Can you work these out from the model? Positions are in its coordinate system, mm. Coordinates: 2 decimals unless noted, no trailing zeros. Loops run counter-clockwise (first coordinate to the right, second up) from the corner with the lowest first, then second, coordinate; pieces in that order, holes last.
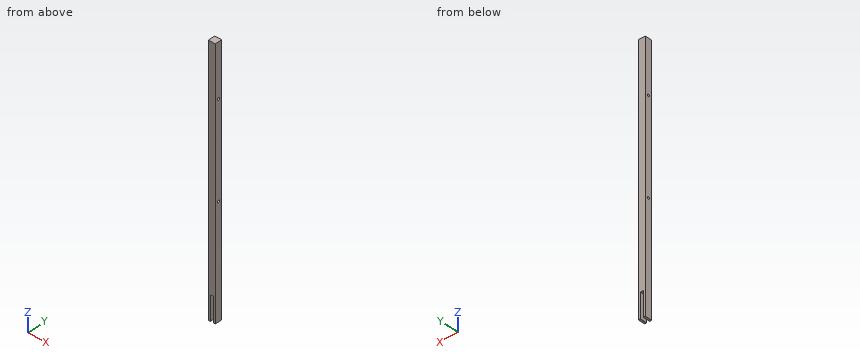
Autodesk Inventor part; units mm, degrees
ref_plane "YZ Plane" through (0, 0, 0) normal (1, 0, 0) x (0, 1, 0)
ref_plane "XZ Plane" through (0, 0, 0) normal (0, 1, 0) x (-1, 0, 0)
ref_plane "XY Plane" through (0, 0, 0) normal (0, 0, 1) x (1, 0, 0)
sketch "Sketch1" plane through (0, 0, 0) normal (0, 0, 1) x (1, 0, 0)
  line L0 (-6, -6) -> (6, -6)
  line L1 (6, -6) -> (6, 6)
  line L2 (6, 6) -> (-6, 6)
  line L3 (-6, 6) -> (-6, -6)
  line L4 (-6, -6) -> (6, 6) construction
  line L5 (6, -6) -> (-6, 6) construction
  point P0 (0, 0)
  dimension "d0" = 12
  dimension "d1" = 12
extrude "Extrusion1" add sketch "Sketch1" along normal blind 440
sketch "Sketch4" plane through (-6, 6, 0) normal (0, 1, 0) x (1, 0, 0)
  line L0 (12, 0) -> (0, 0)
  line L1 (0, 0) -> (0, -440)
  line L2 (12, -440) -> (0, -440)
  line L3 (12, 0) -> (12, -440)
  line L4 (3.5, 0) -> (3.5, -42)
  line L5 (3.5, -42) -> (8.5, -42)
  line L6 (8.5, -42) -> (8.5, 0)
  point P0 (6, 0)
  point P1 (6, -42)
  point P2 (6, 0)
  dimension "d17" = 5
  dimension "d18" = 42
extrude "Extrusion3" cut sketch "Sketch4" against normal through all contours L6 L5 L4 L0
sketch "Sketch5" plane through (6, -6, 0) normal (1, 0, 0) x (0, 0, -1)
  line L0 (-440, 0) -> (-440, 12)
  point P0 (0, 6)
  point P1 (-350, 6)
  point P2 (-189, 6)
  point P3 (-440, 6)
  dimension "d21" = 161
  dimension "d24" = 90
hole "Hole2" at (6, 0, 350) at (6, 0, 189) direction (-1, 0, 0) diameter 4 end through all
equation "\"d0\" = d1"
properties part number "tailboom" material "Balsa"
(1) If I drill on probe 1 along Z at (x, y) = (1.75, 0); probe 2 along Z at (x, y) = (0.25, 0.5); probe 3 along X at (y, z) = (-5, 28), over which ranges is the centre line in solid material (lowest first)?
Check values:
probe 1: z = 42 to 187, 191 to 348, 352 to 440
probe 2: z = 42 to 187.06, 190.94 to 348.06, 351.94 to 440
probe 3: x = -6 to -2.5, 2.5 to 6
(2) I want a section at A-A on y = 0. Write out the boundary of the cut face in (x, z).
Check values:
outline: (-6, 0) - (-2.5, 0) - (-2.5, 42) - (2.5, 42) - (2.5, 0) - (6, 0) - (6, 187) - (-6, 187) - close; (-6, 191) - (6, 191) - (6, 348) - (-6, 348) - close; (-6, 352) - (6, 352) - (6, 440) - (-6, 440) - close
(3) I'm going to push flat-ended pins straight in: pin 1 (5 mm diameter, centred on y = 0, z = 189, fed in from +X); pin 2 (1.5 mm diameter, centred on x = 0.5, y = -2.5, fed in from -Z). Where does each tip first touch, or does it pass through?
Check values:
pin 1: stops at x = 6
pin 2: stops at z = 42
